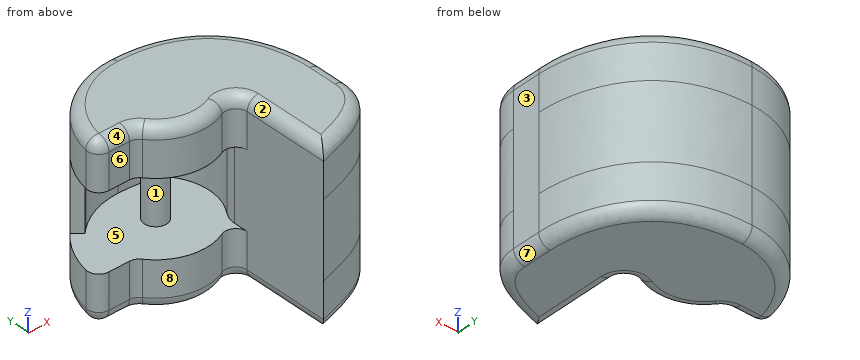
from build123d import *

# Parameters (mm, degrees)
SKETCH1_R            = 2
BOSS_EXTRUDE1_DEPTH  = 8.25
FILLET1_R            = 2
SKETCH1_3_R          = 2
BOSS_EXTRUDE2_DEPTH  = 13.25
FILLET1_OF_MIRROR1_R = 2
BOSS_EXTRUDE3_DEPTH  = 13.25
FILLET5_R            = 4
FILLET6_R            = 2


with BuildPart() as part:
    # Sketch1 → Boss-Extrude1 (new body)
    with BuildSketch(Plane.XY):
        with BuildLine():
            Line((7, -15.5), (7, -25.5))
            add(Edge.make_bspline(
                [(7, -25.5), (10.542331325, -24.196544486), (20, -22.646886742), (20, -15.5)],
                knots=[0, 0, 0, 0, 1, 1, 1, 1], degree=3))
            Line((20, -15.5), (20, -10.5))
            add(Edge.make_bspline(
                [(20, -10.5), (20, -3.471131344), (16.29951196, 9.5), (0, 9.5)],
                knots=[0, 0, 0, 0, 1, 1, 1, 1], degree=3))
            ThreePointArc((0, 9.5), (-10.431323023, 5.282403127), (-15, -5))
            Line((-15, -5), (-8.077747211, -5))
            ThreePointArc((-8.077747211, -5), (-0.892381106, -9.457994288), (7, -6.422616289))
            Line((7, -6.422616289), (7, -15.5))
        make_face()
        Circle(SKETCH1_R, mode=Mode.SUBTRACT)
        Circle(SKETCH1_R)
    boss_extrude1 = extrude(amount=BOSS_EXTRUDE1_DEPTH)

    # Fillet1
    fillet1_edges = [part.edges().sort_by_distance(p)[0] for p in [
        (7, -6.422616289, 4.125),
        (-8.077747211, -5, 4.125),
        (-15, -5, 4.125),
    ]]
    fillet(fillet1_edges, radius=FILLET1_R)

    # Sketch1<3> → Boss-Extrude2 (add)
    with BuildSketch(Plane.XY):
        Circle(SKETCH1_3_R)
    extrude(amount=-BOSS_EXTRUDE2_DEPTH)

    # Mirror1: Boss-Extrude1 across plane
    add(boss_extrude1.mirror(Plane(origin=(0, 0, -6.625), x_dir=(1, 0, 0), z_dir=(0, 0, -1))))

    # Fillet1 of Mirror1
    fillet1_of_mirror1_edges = [part.edges().sort_by_distance(p)[0] for p in [
        (7, -6.422616289, -17.375),
        (-8.077747211, -5, -17.375),
        (-15, -5, -17.375),
    ]]
    fillet(fillet1_of_mirror1_edges, radius=FILLET1_OF_MIRROR1_R)

    # Sketch2 → Boss-Extrude3 (add)
    with BuildSketch(Plane(origin=(0, 0, 0), x_dir=(-1, 0, 0), z_dir=(0, 0, -1))):
        with BuildLine():
            Line((-7, -25.5), (-7, -10.356157589))
            Line((-7, -10.356157589), (-7, -6.892055973))
            ThreePointArc((-7, -6.892055973), (-8.464101615, -8.356157589), (-9, -10.356157589))
            Line((-9, -10.356157589), (-9, -22.771805639))
            add(Edge.make_bspline(
                [(-18, -15.5), (-18, -15.755810099), (-17.96384044, -16.287511283), (-17.769644463, -17.176482985), (-17.326663811, -18.150730827), (-16.473613849, -19.194167826), (-14.905607021, -20.459045473), (-12.82414289, -21.481239618), (-10.597371428, -22.278497003), (-9.539012997, -22.607951452), (-9, -22.771805639)],
                knots=[0, 0, 0, 0, 0.050516154, 0.101032309, 0.202064618, 0.303096927, 0.404129236, 0.606193854, 0.707226163, 0.808258472, 0.808258472, 0.808258472, 0.808258472], degree=3))
            Line((-18, -15.5), (-18, -10.5))
            add(Edge.make_bspline(
                [(-6.962022671, 6.463763635), (-7.052846693, 6.433357714), (-7.813282932, 6.171704453), (-9.764374575, 5.337056232), (-12.300959997, 3.59990947), (-14.595833208, 1.024905795), (-16.245773011, -1.88869544), (-17.142002116, -4.439111746), (-17.608268155, -6.440579265), (-17.843029574, -7.893234579), (-17.952096873, -9.034515744), (-17.993489628, -9.897259581), (-18, -10.296370516), (-18, -10.5)],
                knots=[0.179104723, 0.179104723, 0.179104723, 0.179104723, 0.1875, 0.25, 0.375, 0.5, 0.625, 0.75, 0.8125, 0.875, 0.9375, 0.96875, 1, 1, 1, 1], degree=3))
            ThreePointArc((-6.962022671, 6.463763635), (-3.797646999, 8.707920376), (0, 9.5))
            add(Edge.make_bspline(
                [(0, 9.5), (-16.29951196, 9.5), (-20, -3.471131344), (-20, -10.5)],
                knots=[0, 0, 0, 0, 1, 1, 1, 1], degree=3))
            Line((-20, -10.5), (-20, -15.5))
            add(Edge.make_bspline(
                [(-20, -15.5), (-20, -22.646886742), (-10.542331325, -24.196544486), (-7, -25.5)],
                knots=[0, 0, 0, 0, 1, 1, 1, 1], degree=3))
        make_face()
        with BuildLine():
            ThreePointArc((-9, -10.356157589), (-8.464101615, -8.356157589), (-7, -6.892055973))
            Line((-7, -6.892055973), (-7, -6.422616289))
            ThreePointArc((-7, -6.422616289), (-9.499958745, 0.027997239), (-6.962022671, 6.463763635))
            add(Edge.make_bspline(
                [(-6.962022671, 6.463763635), (-7.052846693, 6.433357714), (-7.813282932, 6.171704453), (-9.764374575, 5.337056232), (-12.300959997, 3.59990947), (-14.595833208, 1.024905795), (-16.245773011, -1.88869544), (-17.142002116, -4.439111746), (-17.608268155, -6.440579265), (-17.843029574, -7.893234579), (-17.952096873, -9.034515744), (-17.993489628, -9.897259581), (-18, -10.296370516), (-18, -10.5)],
                knots=[0.179104723, 0.179104723, 0.179104723, 0.179104723, 0.1875, 0.25, 0.375, 0.5, 0.625, 0.75, 0.8125, 0.875, 0.9375, 0.96875, 1, 1, 1, 1], degree=3))
            Line((-18, -10.5), (-18, -15.5))
            add(Edge.make_bspline(
                [(-18, -15.5), (-18, -15.755810099), (-17.96384044, -16.287511283), (-17.769644463, -17.176482985), (-17.326663811, -18.150730827), (-16.473613849, -19.194167826), (-14.905607021, -20.459045473), (-12.82414289, -21.481239618), (-10.597371428, -22.278497003), (-9.539012997, -22.607951452), (-9, -22.771805639)],
                knots=[0, 0, 0, 0, 0.050516154, 0.101032309, 0.202064618, 0.303096927, 0.404129236, 0.606193854, 0.707226163, 0.808258472, 0.808258472, 0.808258472, 0.808258472], degree=3))
            Line((-9, -22.771805639), (-9, -10.356157589))
        make_face()
        with BuildLine():
            ThreePointArc((0, 9.5), (-3.797646999, 8.707920376), (-6.962022671, 6.463763635))
            add(Edge.make_bspline(
                [(0, 7.5), (-0.46330758, 7.5), (-1.408127817, 7.476315508), (-3.148637138, 7.339831525), (-5.045865316, 7.030251245), (-6.376692574, 6.659719511), (-6.962022671, 6.463763635)],
                knots=[0, 0, 0, 0, 0.03125, 0.0625, 0.125, 0.179104723, 0.179104723, 0.179104723, 0.179104723], degree=3))
            ThreePointArc((0, 7.5), (4.480264496, 6.704136669), (8.41232664, 4.413928013))
            ThreePointArc((8.41232664, 4.413928013), (4.915164488, 8.129646859), (0, 9.5))
        make_face()
        with BuildLine():
            ThreePointArc((10.756875796, 4.957912553), (5.83825606, 8.317928453), (0, 9.5))
            ThreePointArc((0, 9.5), (4.915164488, 8.129646859), (8.41232664, 4.413928013))
            ThreePointArc((8.41232664, 4.413928013), (8.878084444, 3.999472118), (9.323449498, 3.563176359))
            Line((9.323449498, 3.563176359), (10.756875796, 4.957912553))
        make_face()
    extrude(amount=BOSS_EXTRUDE3_DEPTH)

    # Fillet5
    fillet5_edges = [part.edges().sort_by_distance(p)[0] for p in [
        (6.962022671, 6.463763635, -6.625),
        (7, -6.422616289, -6.625),
    ]]
    fillet(fillet5_edges, radius=FILLET5_R)

    # Fillet6
    fillet6_edges = [part.edges().sort_by_distance(p)[0] for p in [
        (15.288594231, -22.445576253, 8.25),
        (20, -13, 8.25),
        (14.507114548, 4.059861745, 8.25),
        (-10.944293973, -5, 8.25),
        (-9.53465116, 6.082286189, 8.25),
        (7, -17.928078794, 8.25),
        (-2.196224683, -9.24265098, 8.25),
        (-14.30901072, -4.270556616, 8.25),
        (6.063219066, -8.662178481, 8.25),
        (-8.239492059, -5.206291187, 8.25),
        (14.507114548, 4.059861745, -21.5),
        (20, -13, -21.5),
        (15.288594231, -22.445576253, -21.5),
        (-9.53465116, 6.082286189, -21.5),
        (-10.944293973, -5, -21.5),
        (7, -17.928078794, -21.5),
        (-2.196224683, -9.24265098, -21.5),
        (-14.30901072, -4.270556616, -21.5),
        (6.063219066, -8.662178481, -21.5),
        (-8.239492059, -5.206291187, -21.5),
    ]]
    fillet(fillet6_edges, radius=FILLET6_R)


solid = part.part
Part model, mm, in its own coordinate system. Face numbers are marked on the shaded views. A direction names the side the tool comes from. Coordinates: 2 decimals unless noted, no trailing zeros.
(1) Pin check, flat tips, straight feed: pin 1 Ø10 at (y, z) = (2, -13) entering from +X; pin 2 Ø4 at (x, z) = (7.5, -4) entering from -Y; pin 3 Ø4 at (x, z) = (15, -12) entering from +Y. Stop position of each tip, or through.
Check sheet entries:
pin 1: stops at x = 18.73
pin 2: stops at y = -25.5
pin 3: stops at y = 5.44
(2) Pull direction Z, two halves, no side cores. Call the marked faces 1, 2 and 3: pulls with the +Z half, pulls with the -Z half, needs draft (parallel to the pull), parting line crosses it, or undercut.
Check sheet entries:
face 1: undercut
face 2: pulls with the +Z half
face 3: needs draft
(3) Tool access for the marked faces 4, 5, 6, 7 and 8: list every direction of +Z, -Z, +X, -X, +Y, -Y with a clear straight run to the whole face (end or side of a thin tool).
Check sheet entries:
face 4: +Z, -X, -Y
face 5: none
face 6: +Z, -Z, -X, -Y
face 7: -Z, +X, +Y, -Y
face 8: +Z, -Z, -Y
(4) Probe L1, parallel to Z at x = -1, y = -5; L2, parallel to X at y = 4.5, z = -12.75; L3, parallel to X at y = -1.5, z = -6.5. List the from-to ranges inside material, lowest first.
Check sheet entries:
L1: z = -21.5 to -13.25, 0 to 8.25
L2: x = -10.29 to -8.31, 8.37 to 14.07
L3: x = -1.32 to 1.32, 9.38 to 18.15
